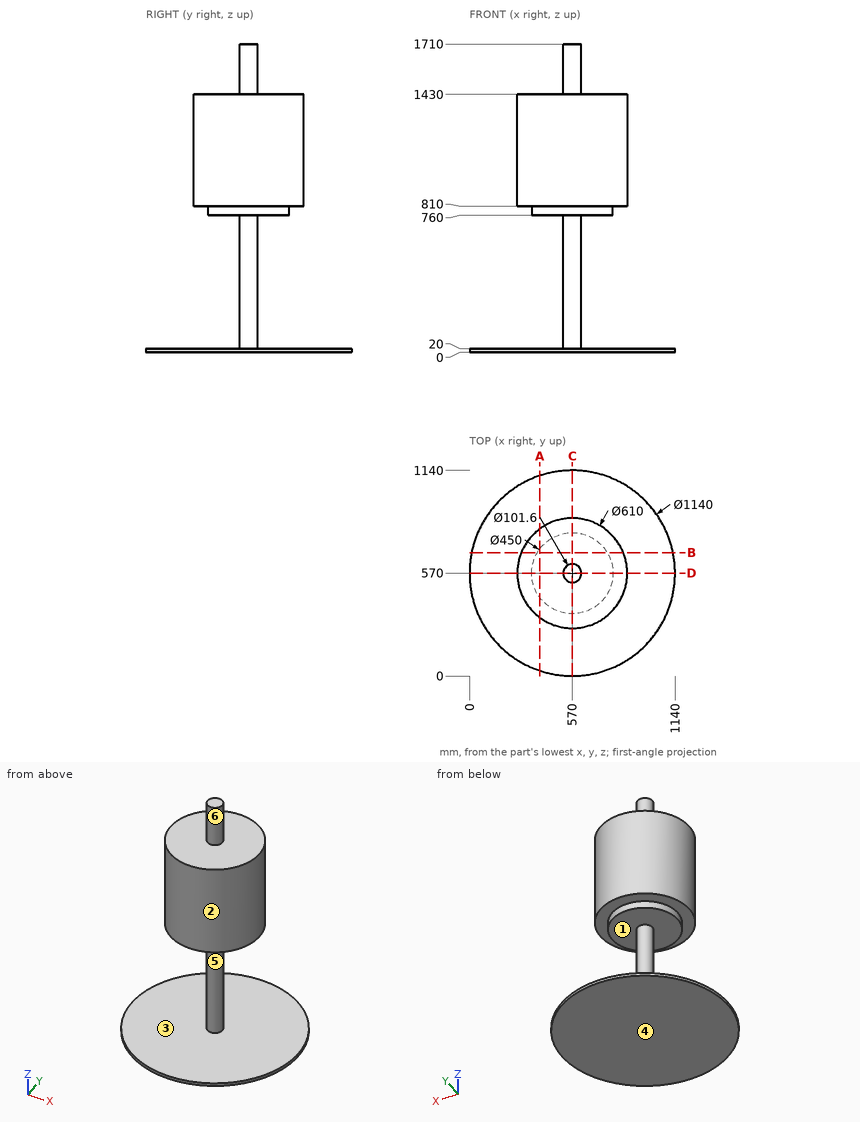
Could you check a few things on this drawing? It's one solid part, dimensions in mm from its lowest x, y, z. A direction names the side the tool comes from. Round coordinates to 2 decimals unless told otherwise and drop trailing zeros. Order: outer loops, then holes, each group sorted by start corner. A loop starts at its lowest first (then second) coordinate and runs counter-clockwise, first axis right, second up. Notation, with made-up numbers: (-4.5, 12.25) -> (22.5, 12.25) arc R26 cw to (22.5, 44.25) -> close; hole circle Ø5 at (5.25, 67). An arc over 180 degrees is marked (long way). One line per question, with ' | ' between items.
Q1. Which directions (+Z, -Z, +X, -X, +Y, -Y) give clear straight access to the entire face, cutting with the end or side of a thin tool? Please do the marked faces 5 and 6.
Computed values:
face 5: none | face 6: +Z
Q2. If we section it at C-C on x = 570: Write out the boundary of the cut face in (y, z).
Computed values:
outline: (0, 0) -> (1140, 0) -> (1140, 20) -> (620.8, 20) -> (620.8, 760) -> (795, 760) -> (795, 810) -> (875, 810) -> (875, 1430) -> (620.8, 1430) -> (620.8, 1710) -> (519.2, 1710) -> (519.2, 1430) -> (265, 1430) -> (265, 810) -> (345, 810) -> (345, 760) -> (519.2, 760) -> (519.2, 20) -> (0, 20) -> close
Q3. If I drill on line 1 (Z direction, x = 786.5, y = 614); line 2 (Z direction, x = 372, y = 949); line 3 (X direction, y = 520.5, z = 1174.5), over which ranges is the centre line in solid material (lowest first)? Write a range as from..to.
Computed values:
line 1: 0..20, 760..1430 | line 2: 0..20 | line 3: 269.04..870.96
Q4. If we section it at B-B on y = 684: Write out the boundary of the cut face in (x, z), plus the area to 3 significant figures.
Computed values:
outline: (11.52, 0) -> (1128.48, 0) -> (1128.48, 20) -> (11.52, 20) -> close; (287.11, 810) -> (376.02, 810) -> (376.02, 760) -> (763.98, 760) -> (763.98, 810) -> (852.89, 810) -> (852.89, 1430) -> (287.11, 1430) -> close | area: 393,000 mm²
Q5. I'm going to push flat-ended pins straight in: pin 1 (10 mm diameter, centred on x = 783, z = 855.5, fed in from -Y); pin 2 (5 mm diameter, centred on x = 491.5, y = 896.5, fed in from +Z); pin 3 (10 mm diameter, centred on x = 265, y = 272, fed in from -Z); pin 4 (10 mm diameter, centred on y = 583.5, z = 736.5, fed in from -X). Where does each tip first touch, or does it pass through?
Computed values:
pin 1: y = 346.93 | pin 2: z = 20 | pin 3: z = 0 | pin 4: x = 519.92
Q6. If we section it at A-A on x = 390: Write out the boundary of the cut face in (y, z), plus the area to 3 significant figures.
Computed values:
outline: (29.17, 0) -> (1110.83, 0) -> (1110.83, 20) -> (29.17, 20) -> close; (323.78, 810) -> (435, 810) -> (435, 760) -> (705, 760) -> (705, 810) -> (816.22, 810) -> (816.22, 1430) -> (323.78, 1430) -> close | area: 340,000 mm²
Q7. We'd pull the mould along Z, two halves only. Please class the marked faces 1, 2, 3 and 4: released by +Z, released by -Z, zero draft, split by the parting line, or undercut.
Computed values:
face 1: undercut | face 2: zero draft | face 3: undercut | face 4: released by -Z
